Model file for the job. Use its own axes, mm. A direction names the side the tool comes from. Give positions to 0.01 mm unless a question says otherwise; leave off trailing zeros. Write each loop counter-clockwise with the first axis right and the second up, starting at its lowest first coordinate (ties: lowest second). Pieces come first, ordered by that corner, then holes. Notation, with made-up numbers: (-24.75, 82.5) - (9.25, 82.5) arc R35 ccw to (9.25, 120.5) - close; hole circle Ø11 at (64.5, 54.25). An arc over 180 degrees is marked (long way). Use a Markdown table: item, result. Add a question column.
```python
from build123d import *

# Parameters (mm, degrees)
BOSS_EXTRUDE1_DEPTH  = 1.65
SKETCH3_W            = 80.7
SKETCH3_H            = 15.9
BOSS_EXTRUDE2_DEPTH  = 13.41
SKETCH4_R            = 1.825
CUT_EXTRUDE1_DEPTH   = 2.65
SKETCH5_W            = 6.15
SKETCH5_H            = 11.05
BOSS_EXTRUDE3_DEPTH  = 12.32
SKETCH6_W            = 4
SKETCH6_H            = 2
BOSS_EXTRUDE4_DEPTH  = 5
CUT_EXTRUDE2_DEPTH   = 11.55
SKETCH8_W            = 27.9
SKETCH8_H            = 11.9
SKETCH8_W_2          = 25.22
SKETCH8_H_2          = 10.05
BOSS_EXTRUDE5_DEPTH  = 5.95
SKETCH9_W            = 10
SKETCH9_H            = 9.66
BOSS_EXTRUDE6_DEPTH  = 1
SKETCH10_W           = 10.5
SKETCH10_H           = 10.16
BOSS_EXTRUDE7_DEPTH  = 14.78
CUT_EXTRUDE3_REACH   = 50.58
SKETCH11_W           = 2.5
SKETCH11_H           = 12.52
SKETCH11_W_2         = 0.825
SKETCH12_R           = 4.275
SKETCH12_R_2         = 4.085
BOSS_EXTRUDE8_DEPTH  = 12.4
SKETCH14_W           = 8.75
SKETCH14_H           = 14.2
BOSS_EXTRUDE9_DEPTH  = 11
SKETCH15_R           = 3.1
SKETCH15_R_2         = 0.8
CUT_EXTRUDE4_DEPTH   = 9.92
CUT_EXTRUDE5_DEPTH   = 10.75
SKETCH18_W           = 8.65
SKETCH18_H           = 4.41
BOSS_EXTRUDE10_DEPTH = 4.64
SKETCH19_W           = 2
SKETCH19_H           = 2
BOSS_EXTRUDE11_DEPTH = 6
SKETCH20_W           = 3.8
SKETCH20_H           = 1.6
BOSS_EXTRUDE12_DEPTH = 0.25


with BuildPart() as part:
    # Sketch1 → Boss-Extrude1 (new body)
    with BuildSketch(Plane(origin=(0, 0, 0), x_dir=(1, 0, 0), z_dir=(0, 1, 0))):
        Polygon((44.75, 44.78), (35, 44.78), (34.13, 45.65), (-34.13, 45.65), (-35, 44.78), (-44.75, 44.78), (-44.75, -45.65), (44.75, -45.65), align=None)
    extrude(amount=BOSS_EXTRUDE1_DEPTH)

    # Sketch3 → Boss-Extrude2 (add)
    with BuildSketch(Plane(origin=(0, 1.65, 0), x_dir=(1, 0, 0), z_dir=(0, 1, 0))):
        with Locations((3.4, -41.12)):
            Rectangle(SKETCH3_W, SKETCH3_H)
    extrude(amount=BOSS_EXTRUDE2_DEPTH)

    # Sketch4 → Cut-Extrude1 (cut, through all)
    with BuildSketch(Plane(origin=(0, 1.65, 0), x_dir=(1, 0, 0), z_dir=(0, 1, 0))):
        with Locations((35.15, 31.38)):
            Circle(SKETCH4_R)
        with Locations((-35.15, 31.38)):
            Circle(SKETCH4_R)
    extrude(amount=-CUT_EXTRUDE1_DEPTH, mode=Mode.SUBTRACT)

    # Sketch5 → Boss-Extrude3 (add)
    with BuildSketch(Plane(origin=(0, 1.65, 0), x_dir=(1, 0, 0), z_dir=(0, 1, 0))):
        with Locations((-41.175, -38.625)):
            Rectangle(SKETCH5_W, SKETCH5_H)
    extrude(amount=BOSS_EXTRUDE3_DEPTH)

    # Sketch6 → Boss-Extrude4 (add)
    with BuildSketch(Plane.XY.offset(44.15)):
        with Locations((-41.175, 4.65)):
            Rectangle(SKETCH6_W, SKETCH6_H)
    extrude(amount=BOSS_EXTRUDE4_DEPTH)

    # Sketch7 → Cut-Extrude2 (cut)
    with BuildSketch(Plane.XY.offset(49.07)):
        Polygon((-34.95, 10.65), (-34.95, 3.65), (-22.75, 3.65), (-22.75, 10.65), (-25.6, 10.65), (-25.6, 12.9), (-32.1, 12.9), (-32.1, 10.65), align=None)
        Polygon((-18.95, 10.65), (-18.95, 3.65), (-6.75, 3.65), (-6.75, 10.65), (-9.6, 10.65), (-9.6, 12.9), (-16.1, 12.9), (-16.1, 10.65), align=None)
        Polygon((-2.95, 10.65), (-2.95, 3.65), (9.25, 3.65), (9.25, 10.65), (6.4, 10.65), (6.4, 12.9), (-0.1, 12.9), (-0.1, 10.65), align=None)
        Polygon((13.05, 10.65), (13.05, 3.65), (25.25, 3.65), (25.25, 10.65), (22.4, 10.65), (22.4, 12.9), (15.9, 12.9), (15.9, 10.65), align=None)
        Polygon((29.05, 10.65), (29.05, 3.65), (41.25, 3.65), (41.25, 10.65), (38.4, 10.65), (38.4, 12.9), (31.9, 12.9), (31.9, 10.65), align=None)
    extrude(amount=-CUT_EXTRUDE2_DEPTH, mode=Mode.SUBTRACT)

    # Sketch8 → Boss-Extrude5 (add)
    with BuildSketch(Plane(origin=(0, 1.65, 0), x_dir=(1, 0, 0), z_dir=(0, 1, 0))):
        with Locations((-27.4, -17.37)):
            Rectangle(SKETCH8_W, SKETCH8_H)
        with Locations((2.35, -17.37)):
            Rectangle(SKETCH8_W, SKETCH8_H)
        with Locations((30.22, -17.37)):
            Rectangle(SKETCH8_W_2, SKETCH8_H_2)
    extrude(amount=BOSS_EXTRUDE5_DEPTH)

    # Sketch9 → Boss-Extrude6 (add)
    with BuildSketch(Plane(origin=(0, 1.65, 0), x_dir=(1, 0, 0), z_dir=(0, 1, 0))):
        with Locations((1.42, 6.37)):
            Rectangle(SKETCH9_W, SKETCH9_H)
    extrude(amount=BOSS_EXTRUDE6_DEPTH)

    # Sketch10 → Boss-Extrude7 (add)
    with BuildSketch(Plane(origin=(0, 2.65, 0), x_dir=(1, 0, 0), z_dir=(0, 1, 0))):
        with Locations((1.42, 6.37)):
            Rectangle(SKETCH10_W, SKETCH10_H)
    extrude(amount=BOSS_EXTRUDE7_DEPTH)

    # Sketch11 → Cut-Extrude3 (cut, up to next)
    with BuildSketch(Plane.ZY.offset(3.83), mode=Mode.PRIVATE) as cut_extrude3_sk1:
        with Locations((-8.205, 11.17)):
            Rectangle(SKETCH11_W, SKETCH11_H)
    cut_extrude3_tool1 = extrude(cut_extrude3_sk1.sketch, amount=-CUT_EXTRUDE3_REACH, mode=Mode.PRIVATE) & part.part
    add(cut_extrude3_tool1.solids().sort_by_distance((-3.83, 11.17, -8.205))[0], mode=Mode.SUBTRACT)
    # Sketch11 → Cut-Extrude3 (cut, up to next)
    with BuildSketch(Plane.ZY.offset(3.83), mode=Mode.PRIVATE) as cut_extrude3_sk2:
        with Locations((-4.535, 11.17)):
            Rectangle(SKETCH11_W, SKETCH11_H)
    cut_extrude3_tool2 = extrude(cut_extrude3_sk2.sketch, amount=-CUT_EXTRUDE3_REACH, mode=Mode.PRIVATE) & part.part
    add(cut_extrude3_tool2.solids().sort_by_distance((-3.83, 11.17, -4.535))[0], mode=Mode.SUBTRACT)
    # Sketch11 → Cut-Extrude3 (cut, up to next)
    with BuildSketch(Plane.ZY.offset(3.83), mode=Mode.PRIVATE) as cut_extrude3_sk3:
        with Locations((-11.0375, 11.17)):
            Rectangle(SKETCH11_W_2, SKETCH11_H)
    cut_extrude3_tool3 = extrude(cut_extrude3_sk3.sketch, amount=-CUT_EXTRUDE3_REACH, mode=Mode.PRIVATE) & part.part
    add(cut_extrude3_tool3.solids().sort_by_distance((-3.83, 11.17, -11.0375))[0], mode=Mode.SUBTRACT)
    # Sketch11 → Cut-Extrude3 (cut, up to next)
    with BuildSketch(Plane.ZY.offset(3.83), mode=Mode.PRIVATE) as cut_extrude3_sk4:
        with Locations((-1.7025, 11.17)):
            Rectangle(SKETCH11_W_2, SKETCH11_H)
    cut_extrude3_tool4 = extrude(cut_extrude3_sk4.sketch, amount=-CUT_EXTRUDE3_REACH, mode=Mode.PRIVATE) & part.part
    add(cut_extrude3_tool4.solids().sort_by_distance((-3.83, 11.17, -1.7025))[0], mode=Mode.SUBTRACT)

    # Sketch12 → Boss-Extrude8 (add)
    with BuildSketch(Plane(origin=(0, 1.65, 0), x_dir=(1, 0, 0), z_dir=(0, 1, 0))):
        with Locations((18.5, 35.65)):
            Circle(SKETCH12_R)
        with Locations((-8.15, 26.15)):
            Circle(SKETCH12_R)
        with Locations((-25.25, 13.9)):
            Circle(SKETCH12_R_2)
    extrude(amount=BOSS_EXTRUDE8_DEPTH)

    # Sketch14 → Boss-Extrude9 (add)
    with BuildSketch(Plane(origin=(0, 1.65, 0), x_dir=(1, 0, 0), z_dir=(0, 1, 0))):
        with Locations((-22.375, 44.14)):
            Rectangle(SKETCH14_W, SKETCH14_H)
    extrude(amount=BOSS_EXTRUDE9_DEPTH)

    # Sketch15 → Cut-Extrude4 (cut)
    with BuildSketch(Plane(origin=(0, 0, -51.24), x_dir=(-1, 0, 0), z_dir=(0, 0, -1))):
        with Locations((22.375, 8.533333602)):
            Circle(SKETCH15_R)
        with Locations((22.375, 8.533333602)):
            Circle(SKETCH15_R_2, mode=Mode.SUBTRACT)
    extrude(amount=-CUT_EXTRUDE4_DEPTH, mode=Mode.SUBTRACT)

    # Sketch17 → Cut-Extrude5 (cut)
    with BuildSketch(Plane.XY.offset(-37.04)):
        with BuildLine():
            Line((-26.375, 8.533333602), (-26.75, 8.533333602))
            Line((-26.75, 8.533333602), (-26.75, 12.65))
            Line((-26.75, 12.65), (-18, 12.65))
            Line((-18, 12.65), (-18, 8.533333602))
            Line((-18, 8.533333602), (-18.375, 8.533333602))
            ThreePointArc((-18.375, 8.533333602), (-22.375, 12.533333602), (-26.375, 8.533333602))
        make_face()
    extrude(amount=-CUT_EXTRUDE5_DEPTH, mode=Mode.SUBTRACT)

    # Sketch18 → Boss-Extrude10 (add)
    with BuildSketch(Plane(origin=(0, 1.65, 0), x_dir=(1, 0, 0), z_dir=(0, 1, 0))):
        with Locations((14.295, 43.695)):
            Rectangle(SKETCH18_W, SKETCH18_H)
    extrude(amount=BOSS_EXTRUDE10_DEPTH)

    # Sketch19 → Boss-Extrude11 (add)
    with BuildSketch(Plane(origin=(0, 0, -45.9), x_dir=(-1, 0, 0), z_dir=(0, 0, -1))):
        with Locations((-13.22, 3.97)):
            Rectangle(SKETCH19_W, SKETCH19_H)
    extrude(amount=BOSS_EXTRUDE11_DEPTH)

    # Sketch20 → Boss-Extrude12 (add)
    with BuildSketch(Plane.XY.offset(49.07)):
        with Locations((-34.365, 11.95)):
            Rectangle(SKETCH20_W, SKETCH20_H)
        with Locations((-23.335, 11.95)):
            Rectangle(SKETCH20_W, SKETCH20_H)
        with Locations((-7.335, 11.95)):
            Rectangle(SKETCH20_W, SKETCH20_H)
        with Locations((-18.365, 11.95)):
            Rectangle(SKETCH20_W, SKETCH20_H)
        with Locations((8.665, 11.95)):
            Rectangle(SKETCH20_W, SKETCH20_H)
        with Locations((-2.365, 11.95)):
            Rectangle(SKETCH20_W, SKETCH20_H)
        with Locations((24.665, 11.95)):
            Rectangle(SKETCH20_W, SKETCH20_H)
        with Locations((13.635, 11.95)):
            Rectangle(SKETCH20_W, SKETCH20_H)
        with Locations((40.665, 11.95)):
            Rectangle(SKETCH20_W, SKETCH20_H)
        with Locations((29.635, 11.95)):
            Rectangle(SKETCH20_W, SKETCH20_H)
    extrude(amount=BOSS_EXTRUDE12_DEPTH)


solid = part.part
```
(1) Flat gauge pins, fed straight in: pin 1 (1.8 mm diameter, centred on y = 12, z = 41.5, fed in from +X); pin 2 (5 mm diameter, centred on x = 25, z = 18.5, fed in from +Y); pin 3 (5 mm diameter, centred on x = 12, y = 6.5, fed in from +Z). Where does each tip first touch, or does it go through?
(2) Probe probe 1 along X at (y, z) = (8, 45); probe 2 along X at (y, z) = (1.2, -31.38) (3 decimals); probe 3 along Z at (x, y) = (-25.5, 9). List the from-to ranges inside material, lowest first. Write a range as [from, to].
(3) Band-saw the part on B-B (z = -13.9). Write the cut outline in (x, y) (3 decimals).
(4) Band-saw the part on A-A (z = -35.65). Write the cut outline in (x, y) (3 decimals).
(5) Which spindle directions (+Z, -Z, +X, -X, +Y, -Y) get a long thin tool onto all of the face, cutting with end or side? Do faces 4 (the flat face through (-22, 7, -37.04)), 5 (the flat face through (-41, 8, 33.1)), 6 (the flat face through (-41, 13.97, 39)), 7 (the flat face through (-9.6, 12, 43)). Say none if no direction does.
(6) Two-plate mould, pull along Y, no slides. Class faces 1 (the flat face through (1, 4.91, -5)), 2 (the flat face through (-44.25, 8, 39)), 3 (the flat face through (-25.6, 12, 43)): +Y half, -Y half, draft (parallel to the pull), parting line (faces both ways), or undercut.
Model answer:
| question | item | result |
|---|---|---|
| 1 | pin 1 | stops at x = 43.75 |
| 1 | pin 2 | stops at y = 7.6 |
| 1 | pin 3 | stops at z = 49.07 |
| 2 | probe 1 | x = [-36.95, -34.95], [-22.75, -18.95], [-6.75, -2.95], [9.25, 13.05], [25.25, 29.05], [41.25, 43.75] |
| 2 | probe 2 | x = [-44.75, -36.975], [-33.325, 33.325], [36.975, 44.75] |
| 2 | probe 3 | z = [-51.24, -37.04], [-17.98, -9.82], [33.17, 37.52] |
| 3 | outline | (-44.75, 0) - (44.75, 0) - (44.75, 1.65) - (-21.165, 1.65) - (-21.165, 14.05) - (-29.335, 14.05) - (-29.335, 1.65) - (-44.75, 1.65) - close |
| 4 | outline | (-44.75, 0) - (44.75, 0) - (44.75, 1.65) - (22.775, 1.65) - (22.775, 14.05) - (14.225, 14.05) - (14.225, 1.65) - (-44.75, 1.65) - close |
| 5 | face 4 | -X, +Y |
| 5 | face 5 | +X, -X, +Y |
| 5 | face 6 | +Z, -Z, -X, +Y |
| 5 | face 7 | +Z |
| 6 | face 1 | +Y half |
| 6 | face 2 | draft |
| 6 | face 3 | undercut |
